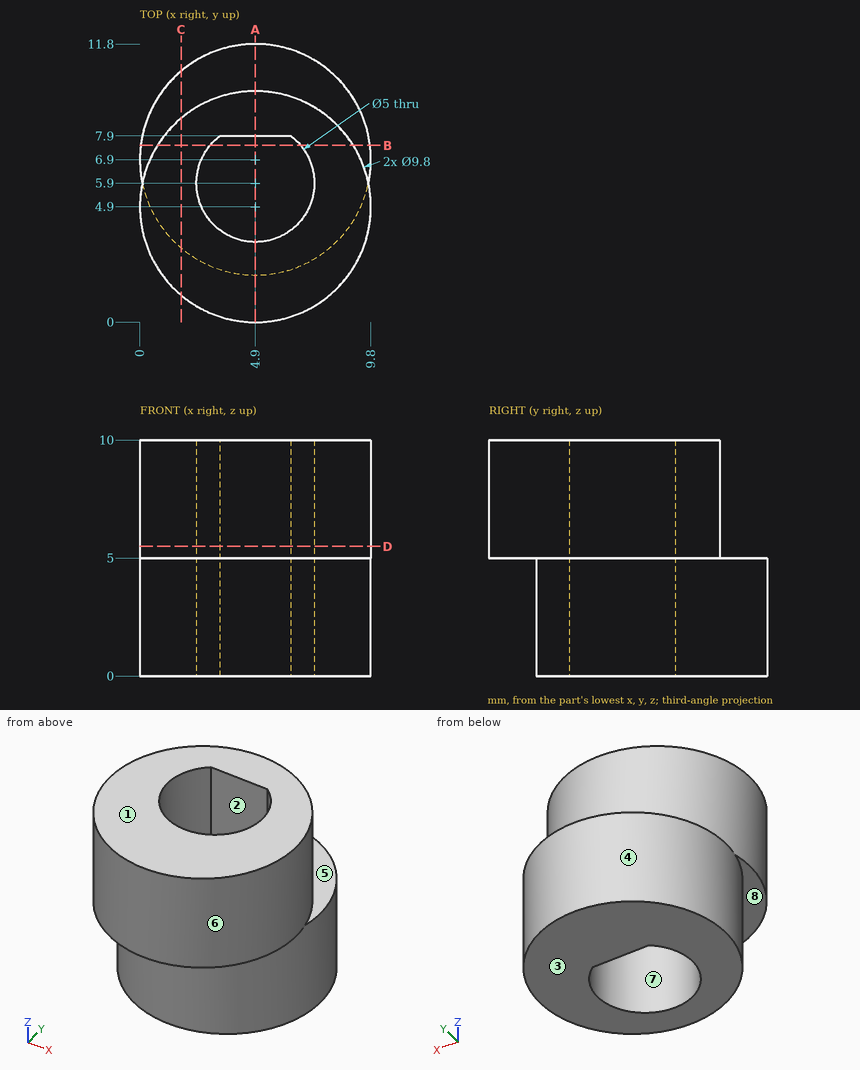
Source: three-view drawing plus pictorial views. Frame: mm from the lowest corner of the part. A direction names the side the tool comes from. Round coordinates to 2 decimals unless told otherwise and drop trailing zeros. Order: outer loops, then holes, each group sorted by start corner. A loop starts at its lowest first (then second) coordinate and runs counter-clockwise, first axis right, second up. Notation, with made-up numbers: M 70.5,48.25 L 116.5,48.25 A29 cw 116.5,80.25 Z; hole C 63,67.25 d10. An arc over 180 degrees is marked long. One line per item, written item: value.
(1) Reachability of the marked faces 1, 2, 3, 4 and 5 from +Z, -Z, +X, -X, +Y, -Y: full face, straight path, thin tool, end or side. Return the list, or none.
Result sheet:
face 1: +Z, +X, -X, +Y, -Y
face 2: +Z, -Z
face 3: -Z, +X, -X, +Y, -Y
face 4: -Z
face 5: +Z, +Y
(2) Pin query (flat end, axial travel): P1, Ø2, axis at x = 8.5, z = 3, coming from the +Y side; P2, Ø1, axis at x = 8, z = 7.5, coming from the -Y side. Return the tip coordinate at first contact, or that it passes through.
Result sheet:
P1: y = 11.05
P2: y = 0.75
(3) Cut plane D-D (z = 5.5). Return the cut outline in (x, y), and give its area (3 significant figures).
Result sheet:
outline: C 4.9,4.9 d9.8; hole M 3.4,7.9 A2.5 ccw long 6.4,7.9 Z
area: 56.8 mm2
(4) Cut plane C-C (x = 1.75). Return the cut outline in (y, z), and give its area (3 significant figures).
Result sheet:
outline: M 1.15,5 L 3.15,5 L 3.15,0 L 10.65,0 L 10.65,5 L 8.65,5 L 8.65,10 L 1.15,10 Z
area: 75.1 mm2
(5) Cut plane B-B (y = 7.5). Return the cut outline in (x, z), and give its area (3 significant figures).
Result sheet:
outline: M 0.04,0 L 2.98,0 L 2.98,10 L 0.75,10 L 0.75,5 L 0.04,5 Z; M 6.82,0 L 9.76,0 L 9.76,5 L 9.05,5 L 9.05,10 L 6.82,10 Z
area: 51.7 mm2
(6) Cut plane A-A (x = 4.9). Return the cut outline in (y, z), and give its area (3 significant figures).
Result sheet:
outline: M 0,5 L 2,5 L 2,0 L 3.4,0 L 3.4,10 L 0,10 Z; M 7.9,0 L 11.8,0 L 11.8,5 L 9.8,5 L 9.8,10 L 7.9,10 Z
area: 53.0 mm2
(7) Pull-direction query (X, two-part tool) for the marked faces 6, 7 and 8; classes: pulls with the +X half, pulls with the -X half, needs draft (parallel to the pull), parting line crosses it, or undercut.
Result sheet:
face 6: parting line crosses it
face 7: undercut
face 8: needs draft
(8) Line query: probe 1 along Y at (x, z) = (4.9, 4.25); probe 2 along Y at (x, z) = (4.9, 5.75); probe 3 along Z at (x, y) = (0.75, 8.75). Output: solid intervals per line, ascending. Write a range as [from, to].
Result sheet:
probe 1: [2, 3.4], [7.9, 11.8]
probe 2: [0, 3.4], [7.9, 9.8]
probe 3: [0, 5]
